Could you check a few things on this model? Use its own coordinates, in mm. Coordinates: 2 decimals unless noted, no trailing zeros. Order: outer loops, then holes, each group sorted by start corner. A loop starts at its lowest first (then second) coordinate and runs counter-clockwise, first axis right, second up. Notation, with made-up numbers: (38, 81.5) -> (51, 81.5) arc R37 cw to (51, 117.5) -> close; hole circle Ø10 at (-31.5, 71). An arc over 180 degrees is marked (long way). Return JSON: item names as keys, results as strings. Group by question number.
from build123d import *

# Parameters (mm, degrees)
F0_W           = 110
F0_H           = 30
F0_R           = 10
F1_DEPTH       = 5
F2_SIZE        = 5
F3_D           = 8.8
F3_CSINK_D     = 17.92
F3_CSINK_ANGLE = 90


with BuildPart() as f1:
    # F0 (on Top) → F1 (new body)
    with BuildSketch(Plane.XY):
        with Locations((55, 15)):
            Rectangle(F0_W, F0_H)
        with Locations((15, 15)):
            Circle(F0_R, mode=Mode.SUBTRACT)
    extrude(amount=F1_DEPTH)

    # F2
    f2_edges = [f1.edges().sort_by_distance(p)[0] for p in [
        (0, 30, 2.5),
        (0, 0, 2.5),
    ]]
    chamfer(f2_edges, length=F2_SIZE)

    # F3 (through all)
    with Locations(Plane(origin=(0, 0, 0), x_dir=(1, 0, 0), z_dir=(0, 0, -1))):
        with Locations((95, -15), (45, -15)):
            CounterSinkHole(F3_D / 2, F3_CSINK_D / 2, counter_sink_angle=F3_CSINK_ANGLE)


solid = f1.part
Q1. We'd pull the mould along X, two halves only. Please class faces 1 (the flat face through (57, 30, 2)), 2 (the conical face through (45.6, 10.42, 4.34)), 3 (the flat face through (3, 28, 2)): pulls with the +X half, pulls with the -X half, needs draft (parallel to the pull), parting line crosses it, or undercut.
Q2. I want a section at A-A on x = 9. Please give me the cut outline in (y, z).
Q3. I want a section at C-C on y = 15. Please give me the cut outline in (x, z).
Q4. I want a section at D-D on x = 45. Please give me the cut outline in (y, z), and give its area (3 significant figures).
Q5. I want a section at B-B on z = 2.5. Please give me the cut outline in (x, y).
Q6. I'm going to push flat-ended pins straight in: pin 1 Ø14 at (x, y) = (45, 15) entering from -Z; pin 2 Ø2 at (y, z) = (27, 2.5) entering from -X. Where does each tip first touch, or does it pass through?
Q7. I need wall thicknesses on line 1 along Y through (x, z) = (45, 4.85); line 2 along Y through (x, z) = (15, 1.5); line 3 along X through (y, z) = (17, 2.05). Which ranges of each line are inside material? Lowest first, please. Write a range as from..to.
Response values:
{
 "1": {"face 1": "needs draft", "face 2": "undercut", "face 3": "pulls with the -X half"},
 "2": {"outline": "(0, 0) -> (7, 0) -> (7, 5) -> (0, 5) -> close; (23, 0) -> (30, 0) -> (30, 5) -> (23, 5) -> close"},
 "3": {"outline": "(0, 0) -> (5, 0) -> (5, 5) -> (0, 5) -> close; (25, 0) -> (36.04, 0) -> (40.6, 4.56) -> (40.6, 5) -> (25, 5) -> close; (49.4, 4.56) -> (53.96, 0) -> (86.04, 0) -> (90.6, 4.56) -> (90.6, 5) -> (49.4, 5) -> close; (99.4, 4.56) -> (103.96, 0) -> (110, 0) -> (110, 5) -> (99.4, 5) -> close"},
 "4": {"outline": "(0, 0) -> (6.04, 0) -> (10.6, 4.56) -> (10.6, 5) -> (0, 5) -> close; (19.4, 4.56) -> (23.96, 0) -> (30, 0) -> (30, 5) -> (19.4, 5) -> close", "area": "85.2 mm²"},
 "5": {"outline": "(0, 5) -> (5, 0) -> (110, 0) -> (110, 30) -> (5, 30) -> (0, 25) -> close; hole circle Ø20 at (15, 15); hole circle Ø12.92 at (45, 15); hole circle Ø12.92 at (95, 15)"},
 "6": {"pin 1": "stops at z = 1.96", "pin 2": "stops at x = 1"},
 "7": {"line 1": "y = 0..10.6, 19.4..30", "line 2": "y = 0..5, 25..30", "line 3": "x = 0..5.2, 24.8..38.39, 51.61..88.39, 101.61..110"}
}
